from build123d import *

# Parameters (mm, degrees)
SKETCH_1_R          = 6
EXTRUDE_1_DEPTH     = 50
SKETCH_2_R          = 4
SKETCH_2_R_2        = 2.5
CUT_EXTRUDE_1_DEPTH = 8
EXTRUDE_START       = 5
SKETCH_3_R          = 2.5
EXTRUDE_2_DEPTH     = 5
FILLET_1_R          = 1.7
SKETCH_4_R          = 0.096106959
CUT_EXTRUDE_2_DEPTH = 5
FILLET_2_R          = 1.2
CHAMFER_1_SIZE      = 0.5


with BuildPart() as part:
    # 草图1 → 凸台-拉伸1 (new body)
    with BuildSketch(Plane(origin=(0, 0, 0), x_dir=(1, 0, 0), z_dir=(0, 1, 0))):
        with Locations(Location((0, 0, 0), (0, 0, 270))):
            Circle(SKETCH_1_R)
    extrude(amount=EXTRUDE_1_DEPTH)

    # 草图2 → 切除-拉伸1 (cut)
    with BuildSketch(Plane(origin=(0, 50, 0), x_dir=(1, 0, 0), z_dir=(0, 1, 0))):
        with Locations(Location((0, 0, 0), (0, 0, 270))):
            Circle(SKETCH_2_R)
        with Locations(Location((0, 0, 0), (0, 0, 270))):
            Circle(SKETCH_2_R_2, mode=Mode.SUBTRACT)
    extrude(amount=-CUT_EXTRUDE_1_DEPTH, mode=Mode.SUBTRACT)

    # 草图3 → 凸台-拉伸2 (add)
    with BuildSketch(Plane(origin=(0, 50, 0), x_dir=(1, 0, 0), z_dir=(0, 1, 0)).offset(EXTRUDE_START)):
        with Locations(Location((0, 0, 0), (0, 0, 270))):
            Circle(SKETCH_3_R)
    extrude(amount=-EXTRUDE_2_DEPTH)

    # 圆角1
    fillet_1_edges = [part.edges().sort_by_distance(p)[0] for p in [
        (0, 55, -2.5),
    ]]
    fillet(fillet_1_edges, radius=FILLET_1_R)

    # 草图4 → 切除-拉伸2 (cut)
    with BuildSketch(Plane(origin=(0, 55, 0), x_dir=(1, 0, 0), z_dir=(0, 1, 0))):
        with Locations(Location((0, 0, 0), (0, 0, 270))):
            Circle(SKETCH_4_R)
    extrude(amount=-CUT_EXTRUDE_2_DEPTH, mode=Mode.SUBTRACT)

    # 圆角2
    fillet_2_edges = [part.edges().sort_by_distance(p)[0] for p in [
        (0, 55, -0.096106959),
    ]]
    fillet(fillet_2_edges, radius=FILLET_2_R)

    # 倒角1
    chamfer_1_edges = [part.edges().sort_by_distance(p)[0] for p in [
        (0, 50, -6),
        (0, 50, -4),
    ]]
    chamfer(chamfer_1_edges, length=CHAMFER_1_SIZE)


solid = part.part
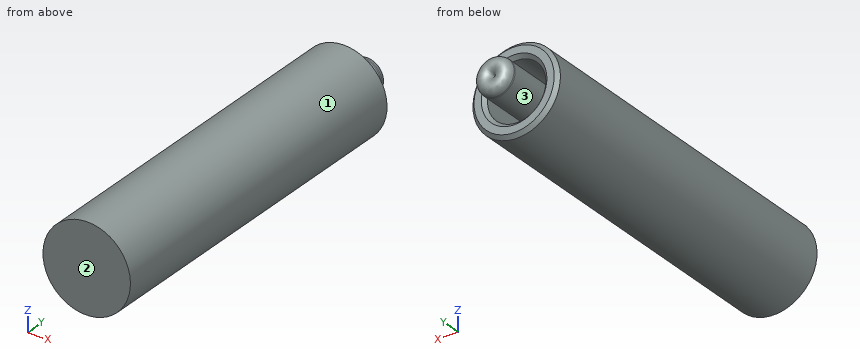
Read the model definition and answer for the solid it produces. Units are mm, in the model's axes. Face numbers are marked on the shaded views. Give positions to 0.01 mm unless a question says otherwise; leave off trailing zeros. Loops run counter-clockwise (first coordinate to the right, second up) from the corner with the lowest first, then second, coordinate; pieces in that order, holes last. Notation, with made-up numbers: (47.25, 25) - (72.25, 25) arc R25 cw to (72.25, 39) - close; hole circle Ø11 at (61.25, 68.5). An arc over 180 degrees is marked (long way). Answer as CSV lines item,"result". Start each with the question number.
1) Each of these flat-tipped pins is pushed along its axis until it touches: pin 1 Ø4 at (y, z) = (31.5, -4) entering from +X; pin 2 Ø4 at (y, z) = (41, -3.5) entering from +X; pin 3 Ø1.5 at (x, y) = (2, 24) entering from -Z. Where does it stop, or does it pass through?
2) Straight lines are drawn through the part: L1, parallel to X at y = 45, z = 0; L2, parallel to Y at x = -3, z = -4; L3, parallel to X at y = 52.4, z = 0. For each, find the intervals that lie inside material, in ascending order. Write a range as from..to.
3) Determine the mould class of the marked faces 1, 2 and 3 for opening direction Z: released by +Z, released by -Z, zero draft, split by the parting line, or undercut.
4) Find section A-A (y = 34). Write down the section's boundary in (x, z).
Findings below:
1,pin 1,"x = 5.66"
1,pin 2,"x = 5.81"
1,pin 3,"z = -5.87"
2,L1,"-6..-4, -2.5..2.5, 4..6"
2,L2,"0..50"
2,L3,"-2.5..-0.1, 0.1..2.5"
3,face 1,"split by the parting line"
3,face 2,"zero draft"
3,face 3,"undercut"
4,outline,"circle Ø12 at (0, 0)"
